Could you check a few things on this model? Use its own coordinates, in mm. A direction names the side the tool comes from. Coordinates: 2 decimals unless noted, no trailing zeros. Loops run counter-clockwise (first coordinate to the right, second up) from the corner with the lowest first, then second, coordinate; pieces in that order, holes last. Notation, with made-up numbers: (-17.75, 81) -> (12.25, 81) arc R25 cw to (12.25, 110) -> close; hole circle Ø9 at (22.5, 59). An arc over 180 degrees is marked (long way). One line per question, with ' | ' between items.
from build123d import *

# Parameters (mm, degrees)
F1_DEPTH     = 4.7625
F3_DEPTH     = 127
F5_DEPTH     = 6.35
F7_DEPTH     = 12.7
F9_DEPTH     = 5.08
F10_T1_DEPTH = 22.563097962
F10_T3_DEPTH = 22.563097962


# Not quite as in the source:
# - a fillet or chamfer that OpenCascade refuses, or shapes differently, is made with other operations: its cross-section is extruded or revolved along the edge and cut away or added
# - a length typed as a fraction of an inch, garbled in the dataset ("3 / 203.2 mm" for 3/8 in), is restored
# - a pattern or mirror of a feature is missing from the dataset's text; its kind, count and spacing are read off the source's solid


with BuildPart() as f1:
    # F0 (on Top) → F1 (new body)
    with BuildSketch(Plane.XY):
        with BuildLine():
            ThreePointArc((-76.2, 0), (0, -76.2), (76.2, 0))
            Line((76.2, 0), (67.31, 0))
            Line((67.31, 0), (67.31, -12.7))
            Line((67.31, -12.7), (-67.31, -12.7))
            Line((-67.31, -12.7), (-67.31, 0))
            Line((-67.31, 0), (-76.2, 0))
        make_face()
    extrude(amount=F1_DEPTH)

    # F2 (on face) → F3 (join)
    with BuildSketch(Plane.XY.offset(4.7625)):
        with BuildLine():
            Line((-67.31, 0), (-76.2, 0))
            ThreePointArc((-76.2, 0), (0, -76.2), (76.2, 0))
            Line((76.2, 0), (67.31, 0))
            ThreePointArc((67.31, 0), (0, -67.31), (-67.31, 0))
        make_face()
    extrude(amount=F3_DEPTH)

    # F4 (on face) → F5 (join)
    with BuildSketch(Plane.XY.offset(131.7625)):
        with BuildLine():
            Line((76.2, 0), (-76.2, 0))
            ThreePointArc((-76.2, 0), (0, -76.2), (76.2, 0))
        make_face()
    extrude(amount=F5_DEPTH)

    # F6 (on face) → F7 (join)
    with BuildSketch(Plane.XY.offset(138.1125)):
        Polygon((12.7, 0), (0, 0), (-12.7, 0), (-12.7, -5.08), (0, -5.08), (12.7, -5.08), align=None)
    extrude(amount=F7_DEPTH)

    # F8 (on face) → F9 (join)
    with BuildSketch(Plane.YZ.offset(12.7)):
        Polygon((-5.08, 150.8125), (-25.4, 138.1125), (-5.08, 138.1125), align=None)
    f9 = extrude(amount=-F9_DEPTH)

    # F9_copies: F9 across plane
    add(f9.mirror(Plane(origin=(0, 0, 0), x_dir=(0, 0, -1), z_dir=(-1, 0, 0))))

    # F10: fillet of radius 5.08 on 2 edges, made by hand

    # F10_s2 → F10_t1 (cut)
    with BuildSketch(Plane.YZ.offset(-21.441548981)):
        with BuildLine():
            ThreePointArc((-6.315469785, 150.0403313843), (-5.0235423361, 150.6156436305), (-3.6230751698, 150.8125))
            Line((-3.6230751698, 150.8125), (-3.6230751698, 150.9141))
            Line((-3.6230751698, 150.9141), (-5.1091384966, 150.9141))
            Line((-5.1091384966, 150.9141), (-6.3693176774, 150.126488012))
            Line((-6.3693176774, 150.126488012), (-6.315469785, 150.0403313843))
        make_face()
    extrude(amount=F10_T1_DEPTH, mode=Mode.SUBTRACT)

    # F10_s4 → F10_t3 (cut)
    with BuildSketch(Plane.YZ.offset(-1.121548981)):
        with BuildLine():
            ThreePointArc((-3.6230751698, 150.8125), (-5.0235423361, 150.6156436305), (-6.315469785, 150.0403313843))
            Line((-6.315469785, 150.0403313843), (-6.3693176774, 150.126488012))
            Line((-6.3693176774, 150.126488012), (-5.1091384966, 150.9141))
            Line((-5.1091384966, 150.9141), (-3.6230751698, 150.9141))
            Line((-3.6230751698, 150.9141), (-3.6230751698, 150.8125))
        make_face()
    extrude(amount=F10_T3_DEPTH, mode=Mode.SUBTRACT)


solid = f1.part
1) On a 3-axis mill with a long thin cutter (end or side, diameter ignored), from which of +Z, -Z, +X, -X, +Y, -Y can I reach the whole of each face in a straight line? I mean faces 4 (the face through (-12.7, -10, 143)), 5 (the face through (1.48, -67.294, 67.374)), 6 (the face through (7.62, -11, 143)), 7 (the face through (1, -12.7, 2)), 8 (the face through (12.7, -10, 143)). Say none if no direction works.
Data:
face 4: +Z, -X, +Y, -Y | face 5: +Y | face 6: +Z, -Y | face 7: -Z, +Y | face 8: +Z, +X, +Y, -Y
2) If we section it at A-A on y = -50.5: Please give me the cut outline in (x, z).
Data:
outline: (-57.06, 0) -> (57.06, 0) -> (57.06, 138.11) -> (-57.06, 138.11) -> close; hole (-44.5, 4.76) -> (44.5, 4.76) -> (44.5, 131.76) -> (-44.5, 131.76) -> close
3) I need wall thicknesses on line 1 along Z through (x, y) = (-43, -51); line 2 along Z through (x, y) = (-21.5, -11); line 3 along X through (y, z) = (-19.5, 70). Which ranges of each line are inside material? Lowest first, please. Write a range as from..to.
Data:
line 1: 0..4.76, 131.76..138.11 | line 2: 131.76..138.11 | line 3: -73.66..-64.42, 64.42..73.66
4) I'm going to push flat-ended pins straight in: pin 1 Ø10 at (y, z) = (-59.5, 69) entering from +X; pin 2 Ø1.4 at (x, z) = (-15, 2) entering from +Y; pin 3 Ø4 at (y, z) = (-7, 2) entering from +X; pin 4 Ø5 at (x, y) = (42.5, -66) entering from -Z. Where does each tip first touch, or does it pass through?
Data:
pin 1: x = 53.26 | pin 2: y = -12.7 | pin 3: x = 76.04 | pin 4: z = 0
5) If we section it at B-B on x = 0: Please give me the cut outline in (y, z), and give its area (3 significant figures).
Data:
outline: (-76.2, 0) -> (-12.7, 0) -> (-12.7, 4.76) -> (-67.31, 4.76) -> (-67.31, 131.76) -> (0, 131.76) -> (0, 150.81) -> (-3.62, 150.81) arc R5.08 ccw to (-5.08, 150.6) -> (-5.08, 138.11) -> (-76.2, 138.11) -> close | area: 1,980 mm²
6) If we section it at D-D on z = 90.5: Please give me the cut outline in (x, y).
Data:
outline: (-76.2, 0) arc R76.2 ccw to (76.2, 0) -> (67.31, 0) arc R67.31 cw to (-67.31, 0) -> close
7) We'd pull the mould along X, two halves only. Please class faces 1 (the face through (-1.68, -76.18, 68.09)), 2 (the face through (-17, 0, 136)), 3 (the face through (-1, -26, 131.762)): pulls with the +X half, pulls with the -X half, needs draft (parallel to the pull), parting line crosses it, or undercut.
Data:
face 1: parting line crosses it | face 2: needs draft | face 3: undercut
8) If we section it at C-C on y = -15: Please give me the cut outline in (x, z), and give its area (3 significant figures).
Data:
outline: (-74.71, 0) -> (74.71, 0) -> (74.71, 138.11) -> (12.7, 138.11) -> (12.7, 144.61) -> (7.62, 144.61) -> (7.62, 138.11) -> (-7.62, 138.11) -> (-7.62, 144.61) -> (-12.7, 144.61) -> (-12.7, 138.11) -> (-74.71, 138.11) -> close; hole (-65.62, 4.76) -> (65.62, 4.76) -> (65.62, 131.76) -> (-65.62, 131.76) -> close | area: 4,040 mm²
